Autodesk Inventor part; units mm, degrees
ref_plane "YZ Plane" through (0, 0, 0) normal (1, 0, 0) x (0, 1, 0)
ref_plane "XZ Plane" through (0, 0, 0) normal (0, 1, 0) x (-1, 0, 0)
ref_plane "XY Plane" through (0, 0, 0) normal (0, 0, 1) x (1, 0, 0)
sketch "Sketch1" plane through (0, 0, 0) normal (0, 1, 0) x (-1, 0, 0)
  line L0 (-16.25, 27) -> (16.25, 27)
  line L1 (16.25, 27) -> (16.25, -27)
  line L2 (16.25, -27) -> (-16.25, -27)
  line L3 (-16.25, -27) -> (-16.25, 27)
  line L4 (-16.25, 27) -> (16.25, -27) construction
  line L5 (16.25, 27) -> (-16.25, -27) construction
  line L6 (16.25, 3) -> (22.25, 3)
  line L7 (22.25, 3) -> (22.25, -3)
  line L8 (22.25, -3) -> (16.25, -3)
  line L9 (16.25, -3) -> (16.25, 3)
  line L10 (-16.25, 3) -> (-22.25, 3)
  line L11 (-22.25, 3) -> (-22.25, -3)
  line L12 (-22.25, -3) -> (-16.25, -3)
  line L13 (-16.25, -3) -> (-16.25, 3)
  circle A0 centre (18.85, 0) radius 1.25
  circle A1 centre (-18.85, 0) radius 1.25
  point P0 (0, 0)
  point P1 (19.25, -3)
  point P2 (19.25, 3)
  point P3 (22.25, 0)
  point P4 (16.25, 0)
  point P5 (-22.25, 0)
  point P6 (-16.25, 0)
  dimension "d0" = 54
  dimension "d1" = 32.5
  dimension "d12" = 6
  dimension "d13" = 6
  dimension "d14" = 6
  dimension "d15" = 6
  dimension "d16" = 2.5
  dimension "d17" = 2.5
  dimension "d18" = 2.6
  dimension "d19" = 37.7
  dimension "d20" = 3
  dimension "d21" = 3
extrude "Extrusion1" add sketch "Sketch1" along normal blind 2
sketch "Sketch2" plane through (0, 2, 0) normal (0, 1, 0) x (1, 0, 0)
  line L0 (-16.25, -27) -> (16.25, -27)
  line L1 (-16.25, 27) -> (-16.25, -27)
  line L2 (16.25, 27) -> (-16.25, 27)
  line L3 (-16.25, -27) -> (-15.25, -27)
  line L4 (-15.25, -27) -> (-15.25, 27)
  line L5 (-15.25, 27) -> (-16.25, 27)
  line L6 (-16.25, 27) -> (-16.25, -27)
  line L7 (0, -27) -> (0, 27) construction
  line L8 (16.25, -27) -> (15.25, -27)
  line L9 (15.25, -27) -> (15.25, 27)
  line L10 (15.25, 27) -> (16.25, 27)
  line L11 (16.25, 27) -> (16.25, -27)
  point P0 (0, 0)
  dimension "d4" = 1
  dimension "d5" = 1
extrude "Extrusion2" add sketch "Sketch2" along normal blind 2 contours L1 L2 L4 L0 | L9 L2 L11 L0
properties part number "Bateria_Podkladka"
CAD build for the part. Positions are in the model's coordinates, mm. A direction names the side the tool comes from. Round coordinates to 2 decimals unless told otherwise and drop trailing zeros. Write each loop counter-clockwise with the first axis right and the second up, starting at its lowest first coordinate (ties: lowest second). Pieces come first, ordered by that corner, then holes. Notation, with made-up numbers: M 11,49.5 L 32,49.5 A13 cw 32,73.5 Z; hole C 40,-34 d7. An arc over 180 degrees is marked long. Use a Markdown table: item, result. Add a question column.
1. 3-axis set-ups, long thin cutter, end or side, ignore diameter. For faces 1 (the face through (0, 2, 0)), 2 (the face through (-19, 1, -3)), 3 (the face through (19, 1, -3)), 4 (the face through (-21, 2, 0)): which of +Z, -Z, +X, -X, +Y, -Y reach the whole face in a straight line?
2. Drill centre lines: probe 1 along X at (y, z) = (2.1, 21); probe 2 along Z at (x, y) = (18.85, 0.8); probe 3 along X at (y, z) = (1.8, 10.5). Where is each one in solid material? Low to high.
3. Slice it at B-B on y = 1.4. Give the cut face in (x, z), then the cut area to 3 significant figures.
4. Slice it at C-C on x = -18.85. Give the cut face in (y, z), then the cut area to 3 significant figures.
5. Slice it at D-D on z = 20.5. Give the cut face in (x, y), then the cut area to 3 significant figures.
6. Flat gauge pins, fed straight in: P1, Ø1.5, axis at y = 1, z = 19, coming from the -X side; P2, Ø4, axis at x = -18.85, z = 0, coming from the +Y side; P3, Ø1, axis at y = 3, z = 8.5, coming from the +X side. Where does each tip first touch, or does it go through?
7. Slice it at A-A on z = 0. Give the cut face in (x, y), then the cut area to 3 significant figures.
8. Pull direction Z, two halves, no side cores. Call faces 5 (the face through (0, 1, -27)), 6 (the face through (17.695, 0.986, 0.479)), 7 (the face through (15.25, 3, 0)): released by +Z, released by -Z, zero draft, split by the parting line, or undercut.
Reply:
| question | item | result |
|---|---|---|
| 1 | face 1 | +Z, -Z, +Y |
| 1 | face 2 | -Z, -X, +Y, -Y |
| 1 | face 3 | -Z, +X, +Y, -Y |
| 1 | face 4 | +Z, -Z, -X, +Y |
| 2 | probe 1 | x = -16.25 to -15.25, 15.25 to 16.25 |
| 2 | probe 2 | z = -3 to -1.25, 1.25 to 3 |
| 2 | probe 3 | x = -16.25 to 16.25 |
| 3 | outline | M -22.25,-3 L -16.25,-3 L -16.25,-27 L 16.25,-27 L 16.25,-3 L 22.25,-3 L 22.25,3 L 16.25,3 L 16.25,27 L -16.25,27 L -16.25,3 L -22.25,3 Z; hole C -18.85,0 d2.5; hole C 18.85,0 d2.5 |
| 3 | area | 1,820 mm^2 |
| 4 | outline | M 0,-3 L 2,-3 L 2,-1.25 L 0,-1.25 Z; M 0,1.25 L 2,1.25 L 2,3 L 0,3 Z |
| 4 | area | 7.00 mm^2 |
| 5 | outline | M -16.25,0 L 16.25,0 L 16.25,4 L 15.25,4 L 15.25,2 L -15.25,2 L -15.25,4 L -16.25,4 Z |
| 5 | area | 69.0 mm^2 |
| 6 | P1 | stops at x = -16.25 |
| 6 | P2 | stops at y = 2 |
| 6 | P3 | stops at x = 16.25 |
| 7 | outline | M -22.25,0 L -20.1,0 L -20.1,2 L -22.25,2 Z; M -17.6,0 L 17.6,0 L 17.6,2 L 16.25,2 L 16.25,4 L 15.25,4 L 15.25,2 L -15.25,2 L -15.25,4 L -16.25,4 L -16.25,2 L -17.6,2 Z; M 20.1,0 L 22.25,0 L 22.25,2 L 20.1,2 Z |
| 7 | area | 83.0 mm^2 |
| 8 | face 5 | released by -Z |
| 8 | face 6 | undercut |
| 8 | face 7 | zero draft |
